Can you work these out from the model? Positions are in its coordinate system, mm. Face numbers are marked on the shaded views. Give positions to 0.01 mm unless a question says otherwise; leave off trailing zeros. Loops run counter-clockwise (first coordinate to the right, second up) from the corner with the lowest first, then second, coordinate; pieces in that order, holes last. Notation, with made-up numbers: (49, -9) - (73, -9) arc R22 cw to (73, 6) - close; hole circle Ø6 at (19.25, 62). An arc over 180 degrees is marked (long way). Answer in a Markdown table with one row per item.
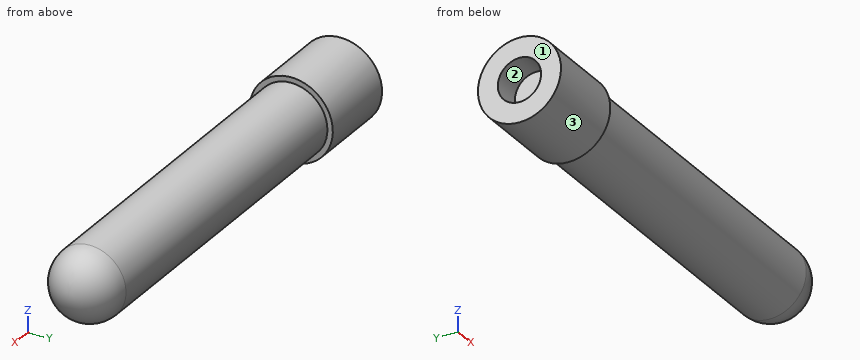
from build123d import *

# Parameters (mm, degrees)
SKETCH_1_R          = 5.75
EXTRUDE_1_DEPTH     = 11.5
SKETCH_3_R          = 5
EXTRUDE_2_DEPTH     = 63.5
FILLET_1_R          = 5
SKETCH_4_R          = 3
CUT_EXTRUDE_1_DEPTH = 4


with BuildPart() as part:
    # 草图1 → 凸台-拉伸1 (new body)
    with BuildSketch(Plane(origin=(0, 0, 0), x_dir=(0, 0, -1), z_dir=(1, 0, 0))):
        Circle(SKETCH_1_R)
    extrude(amount=EXTRUDE_1_DEPTH)

    # 草图3 → 凸台-拉伸2 (add)
    with BuildSketch(Plane.ZY):
        Circle(SKETCH_3_R)
    extrude(amount=-EXTRUDE_2_DEPTH)

    # 圆角1
    fillet_1_edges = [part.edges().sort_by_distance(p)[0] for p in [
        (63.5, 0, -5),
    ]]
    fillet(fillet_1_edges, radius=FILLET_1_R)

    # 草图4 → 切除-拉伸1 (cut)
    with BuildSketch(Plane.ZY):
        Circle(SKETCH_4_R)
    extrude(amount=-CUT_EXTRUDE_1_DEPTH, mode=Mode.SUBTRACT)


solid = part.part
Q1. Imagine slicing it at C-C, the plane x = 28.5. Write out the boundary of the cut face in (y, z), and give its area (3 significant figures).
Checked values:
| item | result |
|---|---|
| outline | circle Ø10 at (0, 0) |
| area | 78.5 mm² |
Q2. If we mould it in two halves opening along Z, with no side actions, what happens to the marked faces 1, 2 and 3? For each: released by +Z, released by -Z, zero draft, split by the parting line, or undercut.
Checked values:
| item | result |
|---|---|
| face 1 | zero draft |
| face 2 | undercut |
| face 3 | split by the parting line |
Q3. Imagine slicing it at A-A, the plane y = 0. Write out the boundary of the cut face in (x, z), and give its area (3 significant figures).
Checked values:
| item | result |
|---|---|
| outline | (0, -5.75) - (11.5, -5.75) - (11.5, -5) - (58.5, -5) arc R5 ccw to (58.5, 5) - (11.5, 5) - (11.5, 5.75) - (0, 5.75) - (0, 3) - (4, 3) - (4, -3) - (0, -3) - close |
| area | 618 mm² |
Q4. If I drill on line 1 (Y direction, x = 2.5, z = 0); line 2 (X direction, y = -4, z = 3.75); line 3 (Z direction, x = 52, y = 4), over which ranges is the centre line in solid material (lowest first)? Write a range as [from, to].
Checked values:
| item | result |
|---|---|
| line 1 | y = [-5.75, -3], [3, 5.75] |
| line 2 | x = [0, 11.5] |
| line 3 | z = [-3, 3] |
Q5. Imagine slicing it at D-D, the plane y = -4. Write out the boundary of the cut face in (x, z).
Checked values:
| item | result |
|---|---|
| outline | (0, -4.13) - (11.5, -4.13) - (11.5, -3) - (58.5, -3) arc R3 ccw to (58.5, 3) - (11.5, 3) - (11.5, 4.13) - (0, 4.13) - close |
Q6. For pin 1 (5 mm diameter, centred on x = 29.5, z = 0, fed in from +Y); pin 2 (6 mm diameter, centred on y = 3, z = 2.5, fed in from +X); pin 3 (5 mm diameter, centred on x = 42.5, z = 1.5, fed in from -Y), each with a flat end and sliding along its axis, tell me the tip position at first contact or that it passes through.
Checked values:
| item | result |
|---|---|
| pin 1 | stops at y = 5 |
| pin 2 | stops at x = 63.42 |
| pin 3 | stops at y = -5 |
